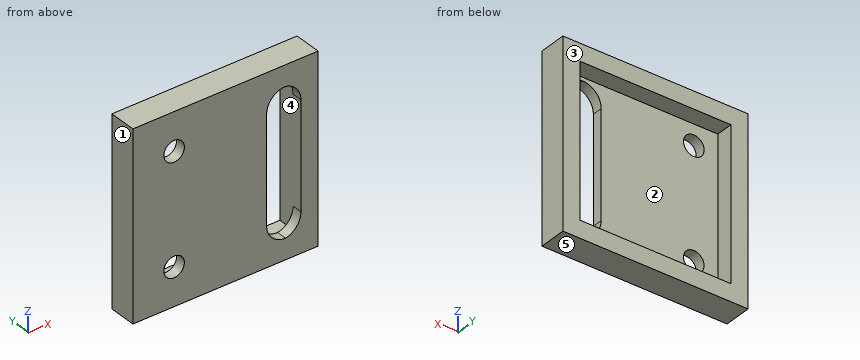
```python
from build123d import *

# Parameters (mm, degrees)
SKETCH2_W           = 27
SKETCH2_H           = 27
BOSS_EXTRUDE1_DEPTH = 4
SKETCH5_W           = 22
SKETCH5_H           = 22
CUT_EXTRUDE2_DEPTH  = 2.5
SKETCH3_R           = 1.5
CUT_EXTRUDE3_DEPTH  = 10
CUT_EXTRUDE4_DEPTH  = 10


with BuildPart() as part:
    # Sketch2 → Boss-Extrude1 (new body)
    with BuildSketch(Plane(origin=(0, 0, 0), x_dir=(1, 0, 0), z_dir=(0, 1, 0))):
        with Locations((13.5, 13.5)):
            Rectangle(SKETCH2_W, SKETCH2_H)
    extrude(amount=BOSS_EXTRUDE1_DEPTH)

    # Sketch5 → Cut-Extrude2 (cut)
    with BuildSketch(Plane(origin=(0, 4, 0), x_dir=(1, 0, 0), z_dir=(0, 1, 0))):
        with Locations((13.5, 13.5)):
            Rectangle(SKETCH5_W, SKETCH5_H)
    extrude(amount=-CUT_EXTRUDE2_DEPTH, mode=Mode.SUBTRACT)

    # Sketch3 → Cut-Extrude3 (cut)
    with BuildSketch(Plane(origin=(0, 0, 0), x_dir=(-1, 0, 0), z_dir=(0, -1, 0))):
        with Locations(Location((-6, 21.5, 0), (0, 0, 90))):
            Circle(SKETCH3_R)
        with Locations(Location((-6, 5.5, 0), (0, 0, 90))):
            Circle(SKETCH3_R)
    extrude(amount=-CUT_EXTRUDE3_DEPTH, mode=Mode.SUBTRACT)

    # Sketch6 → Cut-Extrude4 (cut)
    with BuildSketch(Plane(origin=(0, 1.5, 0), x_dir=(1, 0, 0), z_dir=(0, 1, 0))):
        with BuildLine():
            ThreePointArc((22.25, 24), (20.305456352, 23.194543648), (19.5, 21.25))
            Line((19.5, 21.25), (19.5, 5.75))
            ThreePointArc((19.5, 5.75), (20.305456352, 3.805456352), (22.25, 3))
            ThreePointArc((22.25, 3), (23.865824645, 3.9734162), (24.5, 5.75))
            Line((24.5, 5.75), (24.5, 21.25))
            ThreePointArc((24.5, 21.25), (23.865824645, 23.0265838), (22.25, 24))
        make_face()
    extrude(amount=-CUT_EXTRUDE4_DEPTH, mode=Mode.SUBTRACT)


solid = part.part
```
Source: CAD feature listing. Evaluate the final solid. Frame: model axes, mm. Face numbers are marked on the shaded views. A direction names the side the tool comes from. Give positions to 0.01 mm unless a question says otherwise; leave off trailing zeros. Write each loop counter-clockwise with the first axis right and the second up, starting at its lowest first coordinate (ties: lowest second). Pieces come first, ordered by that corner, then holes.
1. Section query D-D (x = 9.75). Return the cut outline in (y, z), then the cut area to 3 significant figures.
2. First-contact query: pin 1 (6 mm diameter, centred on x = 15, z = -10, fed in from +Y); pin 2 (2.5 mm diameter, centred on x = 6, z = -5.5, fed in from +Y). Flat tips, straight axial feed; report the tip coordinate or a pass-through.
3. Section query B-B (z = -8). Return the cut outline in (x, y).
4. Section query C-C (y = 2.3). Return the cut outline in (x, z).
5. Pull-direction query (X, two-part tool) for the marked faces 1, 2 and 3; classes: +X half, -X half, draft (parallel to the pull), parting line (faces both ways), or undercut.
6. Section query A-A (x = 6). Return the cut outline in (y, z).
7. Access query for the marked faces 4 and 5. Directions: +Z, -Z, +X, -X, +Y, -Y. A direction counts if a zero-diameter tool reaches every point of the face in a straight line with its end or side. Return the directions, or none.
8. Material intervals for line 1 along X through (y, z) = (2.05, -17); line 2 along Z through (x, y) = (17.5, 3.55); line 3 along X through (y, z) = (0.7, -21.5), sorted ascending.
Output values:
1. outline: (0, -27) - (4, -27) - (4, -24.5) - (1.5, -24.5) - (1.5, -2.5) - (4, -2.5) - (4, 0) - (0, 0) - close
1. area: 53.0 mm2
2. pin 1: stops at y = 1.5
2. pin 2: passes through
3. outline: (0, 0) - (19.5, 0) - (19.5, 1.5) - (2.5, 1.5) - (2.5, 4) - (0, 4) - close; (24.5, 0) - (27, 0) - (27, 4) - (24.5, 4) - close
4. outline: (0, -27) - (27, -27) - (27, 0) - (0, 0) - close; hole (2.5, -24.5) - (24.5, -24.5) - (24.5, -2.5) - (2.5, -2.5) - close
5. face 1: -X half
5. face 2: undercut
5. face 3: draft
6. outline: (0, -27) - (4, -27) - (4, -24.5) - (1.5, -24.5) - (1.5, -23) - (0, -23) - close; (0, -20) - (1.5, -20) - (1.5, -7) - (0, -7) - close; (0, -4) - (1.5, -4) - (1.5, -2.5) - (4, -2.5) - (4, 0) - (0, 0) - close
7. face 4: +Y
7. face 5: -Z, +X, -X, +Y, -Y
8. line 1: x = 0 to 2.5, 24.5 to 27
8. line 2: z = -27 to -24.5, -2.5 to 0
8. line 3: x = 0 to 4.5, 7.5 to 19.51, 24.49 to 27
